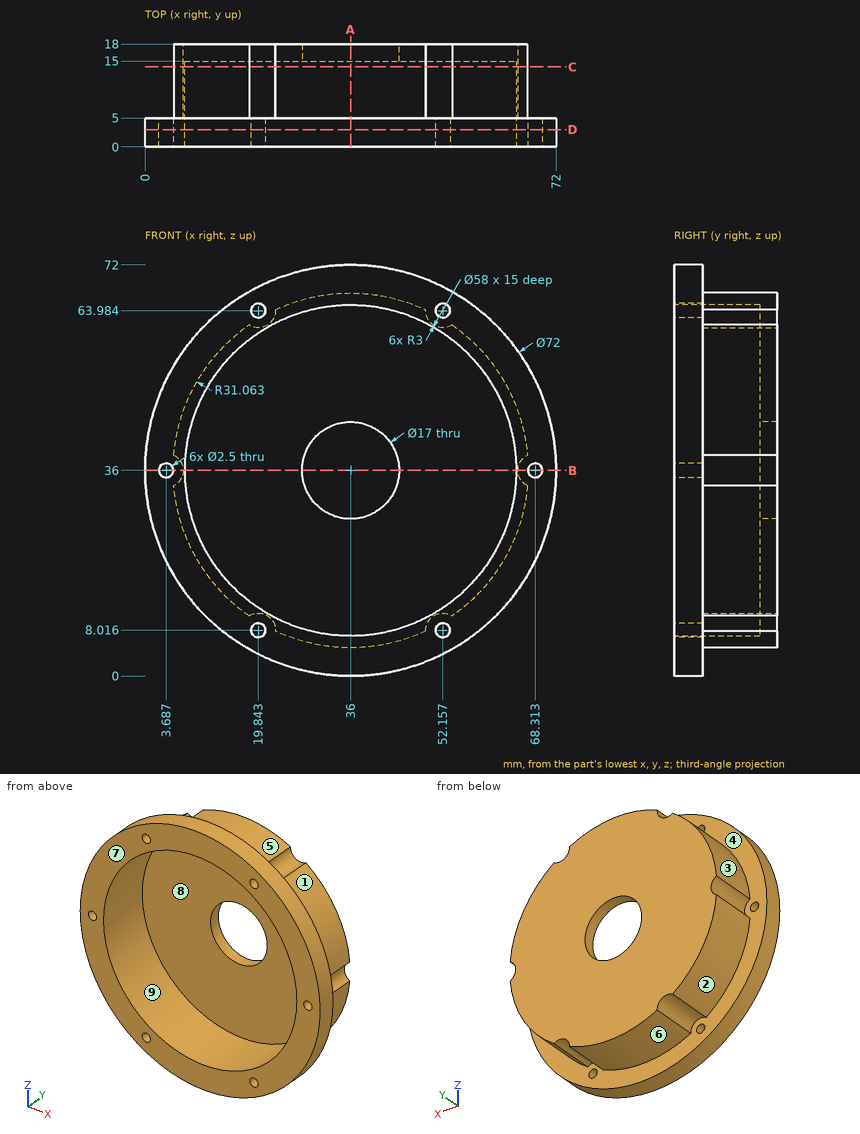
Study the drawing (mm; zero at the part's minimum x, y, z) and answer. A direction names the side the tool comes from. Coordinates: 2 decimals unless noted, no trailing zeros. Order: outer loops, then holes, each group sorted by start corner. A loop starts at its lowest first (then second) coordinate and runs counter-clockwise, first axis right, second up. Notation, with made-up numbers: M 10,53.25 L 51,53.25 A13 cw 51,73.25 Z; hole C 54,-1 d6. An arc over 180 degrees is marked long. Answer as a JSON object with one key per item and string values. Group by question number.
1. Section D-D on y = 3 is taken. Write down the section's boundary in (x, z).
2. Flat-ended cylindrical pins translate along their axes: P1, Ø6, axis at y = 11.5, z = 53.5, coming from the -X side; P2, Ø2, axis at x = 52.16, z = 63.98, coming from the -Y side; P3, Ø1.5, axis at y = 5, z = 51.5, coming from the -X side; P4, Ø6, axis at y = 10.5, z = 53.5, coming from the +X side. Find the tip coordinate at first contact, or state that the pin passes through.
3. Determine the mould class of the marked faces 6, 7, 8 and 9 for opening direction Z: released by +Z, released by -Z, zero draft, split by the parting line, or undercut.
4. Straight lines are drawn through the part: line 1 (X direction, y = 12, z = 56) (1 decimal); line 2 (Y direction, x = 17.5, z = 63); line 3 (Y direction, x = 61.5, z = 26.5). For each, find the intervals that lie inside material, in ascending order.
5. Section A-A on x = 36 is taken. Write down the section's boundary in (y, z).
6. A tool of negligible diameter and unlimited length cuts with its end or side. For the marked faces 1, 2, 3, 4 and 5, from which of +Z, -Z, +X, -X, +Y, -Y can it reach the whole face along a straight path? Write none if from no direction.
7. Section C-C on y = 14 is taken. Write down the section's boundary in (x, z) (1 decimal).
8. Section B-B on z = 36 is taken. Write down the section's boundary in (x, y).
Values follow:
{
 "1": {"outline": "C 36,36 d72; hole C 3.69,36 d2.5; hole C 36,36 d58; hole C 19.84,8.02 d2.5; hole C 19.84,63.98 d2.5; hole C 52.16,8.02 d2.5; hole C 52.16,63.98 d2.5; hole C 68.31,36 d2.5"},
 "2": {"P1": "x = 8.53", "P2": "through", "P3": "x = 3.16", "P4": "x = 63.47"},
 "3": {"face 6": "released by -Z", "face 7": "zero draft", "face 8": "undercut", "face 9": "undercut"},
 "4": {"line 1": "12.2 to 15, 57 to 59.8", "line 2": "0 to 5", "line 3": "15 to 18"},
 "5": {"outline": "M 0,0 L 5,0 L 5,4.94 L 18,4.94 L 18,27.5 L 15,27.5 L 15,7 L 0,7 Z; M 0,65 L 15,65 L 15,44.5 L 18,44.5 L 18,67.06 L 5,67.06 L 5,72 L 0,72 Z"},
 "6": {"face 1": "+Z, +X, +Y", "face 2": "-Z, -X, +Y", "face 3": "+Z, -X, +Y", "face 4": "+Y", "face 5": "+Z, +Y"},
 "7": {"outline": "M 5.1,33.3 A31.1 ccw 18.2,10.5 A3 cw 22.8,7.9 A31.1 ccw 49.2,7.9 A3 cw 53.8,10.5 A31.1 ccw 66.9,33.3 A3 cw 66.9,38.7 A31.1 ccw 53.8,61.5 A3 cw 49.2,64.1 A31.1 ccw 22.8,64.1 A3 cw 18.2,61.5 A31.1 ccw 5.1,38.7 A3 cw Z; hole C 36,36 d58"},
 "8": {"outline": "M 0,0 L 2.44,0 L 2.44,5 L 0,5 Z; M 4.94,0 L 7,0 L 7,15 L 27.5,15 L 27.5,18 L 6.69,18 L 6.69,5 L 4.94,5 Z; M 44.5,15 L 65,15 L 65,0 L 67.06,0 L 67.06,5 L 65.31,5 L 65.31,18 L 44.5,18 Z; M 69.56,0 L 72,0 L 72,5 L 69.56,5 Z"}
}
